Geometry check sheet. Reference: the model listing, model coordinates, mm. Coordinates: 2 decimals unless noted, no trailing zeros.
from build123d import *

# Parameters (mm, degrees)
F0_R     = 3.175
F0_R_2   = 3.571875
F0_R_3   = 3.96875
F0_R_4   = 4.365625
F0_R_5   = 2.778125
F0_R_6   = 2.38125
F0_R_7   = 4.7625
F0_R_8   = 5.159375
F0_R_9   = 1.984375
F0_R_10  = 1.5875
F0_R_11  = 5.55625
F0_R_12  = 6.35
F1_DEPTH = 3.175


with BuildPart() as f1:
    # F0 (on Top) → F1 (new body)
    with BuildSketch(Plane.XY):
        with BuildLine():
            ThreePointArc((0, 63.5), (-31.75, 31.75), (0, 0))
            Line((0, 0), (114.3, 0))
            ThreePointArc((114.3, 0), (118.790128, 1.859872), (120.65, 6.35))
            Line((120.65, 6.35), (120.65, 57.15))
            ThreePointArc((120.65, 57.15), (118.790128, 61.640128), (114.3, 63.5))
            Line((114.3, 63.5), (0, 63.5))
        make_face()
        with Locations((-17.970501, 32.004002)):
            Circle(F0_R, mode=Mode.SUBTRACT)
        with Locations((6.35, 12.7)):
            Circle(F0_R_2, mode=Mode.SUBTRACT)
        with Locations((6.100903, 50.8)):
            Circle(F0_R_3, mode=Mode.SUBTRACT)
        with Locations((25.150903, 50.8)):
            Circle(F0_R_4, mode=Mode.SUBTRACT)
        with Locations((25.4, 12.7)):
            Circle(F0_R, mode=Mode.SUBTRACT)
        with Locations((44.45, 12.7)):
            Circle(F0_R_5, mode=Mode.SUBTRACT)
        with Locations((63.5, 12.7)):
            Circle(F0_R_6, mode=Mode.SUBTRACT)
        with Locations((44.45, 50.8)):
            Circle(F0_R_7, mode=Mode.SUBTRACT)
        with Locations((63.5, 50.8)):
            Circle(F0_R_8, mode=Mode.SUBTRACT)
        with Locations((82.55, 12.7)):
            Circle(F0_R_9, mode=Mode.SUBTRACT)
        with Locations((101.6, 12.7)):
            Circle(F0_R_10, mode=Mode.SUBTRACT)
        with Locations((82.55, 50.8)):
            Circle(F0_R_11, mode=Mode.SUBTRACT)
        with Locations((101.6, 50.8)):
            Circle(F0_R_12, mode=Mode.SUBTRACT)
    extrude(amount=F1_DEPTH)


solid = f1.part
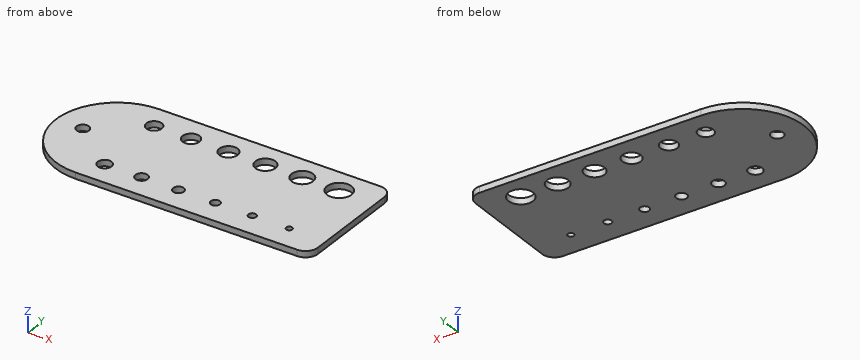
1) Depth check by flat-ended pin: pin 1 (4.5 mm diameter, centred on x = 44.45, y = 12.7, fed in from +Z); pin 2 (15 mm diameter, centred on x = 44.45, y = 50.8, fed in from -Z). Enter the tip coordinate at first touch or a pass-through.
Data:
pin 1: passes through
pin 2: stops at z = 0
2) Section check A-A on x = 101.6. Count the separate pieces of the cut face and the enclosed holes in it, and give its area (3 significant figures).
Data:
separate pieces: 3
enclosed holes: 0
area: 151 mm2
3) Material ranges on probe 1 along Y at (x, z) = (25.4, 1.8) (3 decimals); probe 2 along Y at (x, z) = (44.45, 1.7); probe 3 along X at (y, z) = (34, 2.3), recorded low to high.
Data:
probe 1: y = 0 to 9.525, 15.875 to 46.441, 55.159 to 63.5
probe 2: y = 0 to 9.92, 15.48 to 46.04, 55.56 to 63.5
probe 3: x = -31.67 to -20.44, -15.5 to 120.65
